Build history of the part. All positions in model axes, mm. Round coordinates to 2 decimals unless told otherwise and drop trailing zeros. Write each loop counter-clockwise with the first axis right and the second up, starting at its lowest first coordinate (ties: lowest second). Pieces come first, ordered by that corner, then holes.
Item 1: Band-saw the part on A-A, the plane y = -16.5. Write the cut outline in (x, z).
Item 2: Band-saw the part on B-B, the plane z = -10. Count the separate pieces of the cut face and the enclosed holes in it, then the cut area to 3 significant figures.
Item 3: Band-saw the part on C-C, the plane y = -32.5. Write the cut outline in (x, z).
Item 4: Drop a flat-ended pin along its axis: pin 1 Ø1 at (x, z) = (6, 6.5) entering from +Y. Give the stop position or say it passes through.
Item 5: Wall check: probe 1 along Y at (x, z) = (7, -10); probe 2 along Y at (x, z) = (9.25, -7); probe 3 along Z at (x, y) = (2.25, -32.5). Give the ranges that are in metal, low to high.
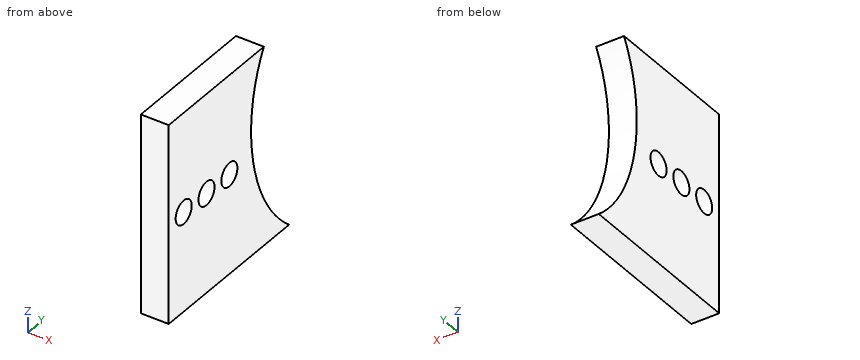
```python
from build123d import *

# Parameters (mm, degrees)
SKETCH1_R           = 4.221837906
BOSS_EXTRUDE1_DEPTH = 10


with BuildPart() as part:
    # Sketch1 → Boss-Extrude1 (new body)
    with BuildSketch(Plane(origin=(0, 0, 0), x_dir=(0, 0, -1), z_dir=(1, 0, 0))):
        with BuildLine():
            Line((-29.05259943, -0.165516433), (-29.05259943, -50.165516433))
            Line((-29.05259943, -50.165516433), (42.210436172, -50.165516433))
            Line((42.210436172, -50.165516433), (42.210436172, 13.142555632))
            add(Edge.make_bspline(
                [(-29.05259943, -0.165516433), (-6.499992704, -12.774809737), (25.427672134, -7.094962856), (42.210436172, 13.142555632)],
                knots=[0, 0, 0, 0, 1, 1, 1, 1], degree=3))
        make_face()
        with Locations((6.578918371, -42.29705463)):
            Circle(SKETCH1_R, mode=Mode.SUBTRACT)
        with Locations((6.578918371, -30.29705463)):
            Circle(SKETCH1_R, mode=Mode.SUBTRACT)
        with Locations((6.578918371, -18.29705463)):
            Circle(SKETCH1_R, mode=Mode.SUBTRACT)
    extrude(amount=BOSS_EXTRUDE1_DEPTH)


solid = part.part
```
Results:
1. outline: (0, -42.21) - (10, -42.21) - (10, -10.4) - (0, -10.4) - close; (0, -2.76) - (10, -2.76) - (10, 29.05) - (0, 29.05) - close
2. separate pieces: 4
2. enclosed holes: 0
2. area: 297 mm2
3. outline: (0, -42.21) - (10, -42.21) - (10, -10.18) - (0, -10.18) - close; (0, -2.98) - (10, -2.98) - (10, 29.05) - (0, 29.05) - close
4. pin 1: stops at y = -6.67
5. probe 1: y = -50.17 to -44.77, -39.82 to -32.77, -27.82 to -20.77, -15.82 to -5.58
5. probe 2: y = -50.17 to -46.5, -38.1 to -34.5, -26.1 to -22.5, -14.1 to -6.12
5. probe 3: z = -42.21 to -10.18, -2.98 to 29.05
